Read the model definition and answer for the solid it produces. Units are mm, in the model's axes. Face numbers are marked on the shaded views. Coordinates: 2 decimals unless noted, no trailing zeros. Loops run counter-clockwise (first coordinate to the right, second up) from the corner with the lowest first, then second, coordinate; pieces in that order, holes last.
from build123d import *

# Parameters (mm, degrees)
F1_DEPTH      = 100
F3_DEPTH      = 98.6
F5_DEPTH      = 90.4
F5_DEPTH_BACK = 126
F7_R          = 1.588882932
F8_DEPTH      = 43
F9_R          = 23
F10_DEPTH     = 1
F10_FACE_R    = 23
F6_R          = 35.9732862146


with BuildPart() as f1:
    # F0 (on Top) → F1 (new body)
    with BuildSketch(Plane.XY):
        with BuildLine():
            Line((-72.5, -20), (72.5, -20))
            ThreePointArc((72.5, -20), (86.678490298, 16.4571509702), (80, 55))
            ThreePointArc((80, 55), (72.5, 58.3856217223), (65, 55))
            ThreePointArc((65, 55), (59.6251005185, 44.7536715994), (57.25, 33.4295518696))
            Line((57.25, 33.4295518696), (57.25, 20))
            Line((57.25, 20), (52.2593490829, 20))
            Line((52.2593490829, 20), (-57.25, 20))
            Line((-57.25, 20), (-57.25, 30.6907939249))
            ThreePointArc((-57.25, 30.6907939249), (-59.2343780506, 43.4481447471), (-65, 55))
            ThreePointArc((-65, 55), (-72.5, 58.3856217223), (-80, 55))
            ThreePointArc((-80, 55), (-88.7033607571, 16.2546639243), (-72.5, -20))
        make_face()
    extrude(amount=F1_DEPTH)

    # F2 (on face) → F3 (cut)
    with BuildSketch(Plane.XZ.offset(20)):
        with BuildLine():
            ThreePointArc((-57.4272125959, 90.5), (-41.3839754635, 92.9294628197), (-26.7793443054, 100))
            Line((-26.7793443054, 100), (-94.0743684769, 100))
            Line((-94.0743684769, 100), (-90.0195017457, 81))
            ThreePointArc((-90.0195017457, 81), (-74.4015116391, 88.0765901597), (-57.4272125959, 90.5))
        make_face()
        with BuildLine():
            Line((90.444765985, 100), (26.7793443054, 100))
            ThreePointArc((26.7793443054, 100), (41.3839754635, 92.9294628197), (57.4272125959, 90.5))
            ThreePointArc((57.4272125959, 90.5), (74.4015116391, 88.0765901597), (90.0195017457, 81))
            Line((90.0195017457, 81), (90.444765985, 100))
        make_face()
    extrude(amount=-F3_DEPTH, mode=Mode.SUBTRACT)

    # F4 (on Right) → F5 (cut, two sides)
    with BuildSketch(Plane.YZ) as f5_sk:
        with BuildLine():
            ThreePointArc((24.7983019799, 91.6626080871), (46.3463766624, 84.825875611), (66.7543932796, 75.1009956002))
            Line((66.7543932796, 75.1009956002), (66.7543932796, 98.7012907863))
            Line((66.7543932796, 98.7012907863), (24.7983019799, 98.7012907863))
            Line((24.7983019799, 98.7012907863), (24.7983019799, 91.6626080871))
        make_face()
    extrude(amount=-F5_DEPTH, mode=Mode.SUBTRACT)
    extrude(f5_sk.sketch, amount=F5_DEPTH_BACK, mode=Mode.SUBTRACT)

    # F7 (on face) → F8 (join)
    with BuildSketch(Plane(origin=(0, 20, 0), x_dir=(-1, 0, 0), z_dir=(0, 1, 0))):
        with Locations((0, 40.5010841787)):
            Circle(F7_R)
    extrude(amount=F8_DEPTH)

    # F9 (on face) → F10 (join)
    with BuildSketch(Plane(origin=(0, 63, 0), x_dir=(-1, 0, 0), z_dir=(0, 1, 0))):
        with Locations((0, 40.5010841787)):
            Circle(F9_R)
    extrude(amount=F10_DEPTH)

    # F10_face (on face) → F11 section 0
    with BuildSketch(Plane(origin=(0, 64, 40.5010841787), x_dir=(-1, 0, 0), z_dir=(0, 1, 0))):
        Circle(F10_FACE_R)
    # F6 (on face) → F11 section 1
    with BuildSketch(Plane(origin=(0, 20, 0), x_dir=(-1, 0, 0), z_dir=(0, 1, 0))):
        with Locations((0, 40.5)):
            Circle(F6_R)
    loft()


solid = f1.part
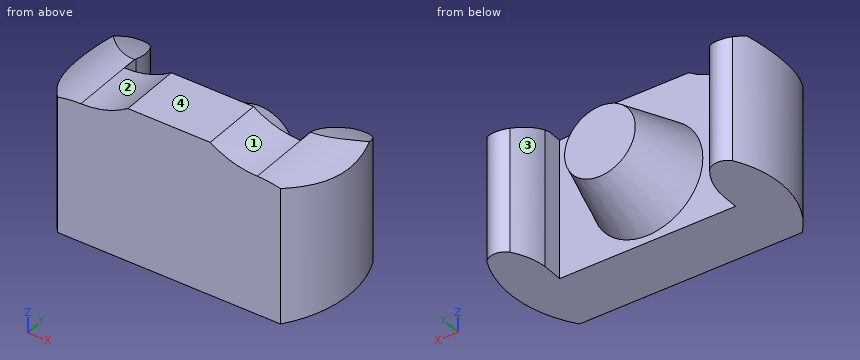
Q1. Straight lines are drawn through the part: probe 1 along X at (y, z) = (44.5, 34.5); probe 2 along Y at (x, z) = (-42.5, 36); probe 3 along X at (y, z) = (37, 57). For each, find the intervals that lie inside material, in ascending order.
Findings below:
probe 1: x = -85.06 to -59.59, -28.12 to 28.12, 59.53 to 84.02
probe 2: y = -20 to 20
probe 3: x = -87.33 to -57.73, -26.2 to 26.2, 57.65 to 85.82
Q2. A cutting plane is placed at B-B (x = 76). Give the vertices of the cut face in (y, z).
Findings below:
outline: (-14.88, 0) - (57.75, 0) - (57.75, 79.82) arc R164.59 ccw to (38.82, 87.59) - (-14.88, 87.59) - close
Q3. A cutting plane is placed at C-C (y = 23). Count the separate pieces of the cut face and the enclosed holes in it, then the cut area to 3 significant figures.
Findings below:
separate pieces: 3
enclosed holes: 0
area: 9,270 mm2
Q4. Determine the mould class of the marked faces 1, 2, 3 and 4 for opening direction X: +X half, -X half, draft (parallel to the pull), parting line (faces both ways), or undercut.
Findings below:
face 1: +X half
face 2: -X half
face 3: undercut
face 4: draft
Q5. A cutting plane is placed at D-D (x = -77). Give the vertices of the cut face in (y, z), then the cut area to 3 significant figures.
Findings below:
outline: (-14.49, 0) - (57.32, 0) - (57.32, 80.03) arc R164.59 ccw to (39.79, 87.26) - (-14.49, 87.26) - close
area: 6,210 mm2
Q6. Flat-ended cylindrical pins translate along their axes: pin 1 Ø5 at (y, z) = (15.5, 68) entering from -X; pin 2 Ø1.5 at (y, z) = (44.5, 73.5) entering from -X; pin 3 Ø6.5 at (y, z) = (29.5, 24.5) entering from -X. Find the tip coordinate at first contact, or state that the pin passes through.
Findings below:
pin 1: stops at x = -88.85
pin 2: stops at x = -85.33
pin 3: stops at x = -88.91
Q7. A cutting plane is placed at A-A (y = -3.5). Give the vertices of the cut face in (x, z).
Findings below:
outline: (-83.39, 0) - (81.78, 0) - (81.78, 85.4) arc R60.66 ccw to (57.43, 90.5) arc R54.19 cw to (26.78, 100) - (-26.78, 100) arc R54.19 cw to (-57.43, 90.5) arc R60.66 ccw to (-83.39, 84.66) - close
